from build123d import *

# Parameters (mm, degrees)
BOSS_EXTRUDE1_DEPTH      = 381
BOSS_EXTRUDE1_DEPTH_BACK = 381
SKETCH1_W                = 12.7
SKETCH1_H                = 12.7
SKETCH1_W_2              = 9.525
SKETCH1_H_2              = 9.525


with BuildPart() as part:
    # Sketch1 → Boss-Extrude1 (new, two sides: drawn at the far end of the back side and taken through both)
    with BuildSketch(Plane.XY.offset(-BOSS_EXTRUDE1_DEPTH_BACK)):
        with Locations((323.85, 95.25)):
            Rectangle(SKETCH1_W, SKETCH1_H)
        with Locations((323.85, 95.25)):
            Rectangle(SKETCH1_W_2, SKETCH1_H_2, mode=Mode.SUBTRACT)
    extrude(amount=BOSS_EXTRUDE1_DEPTH + BOSS_EXTRUDE1_DEPTH_BACK)


solid = part.part
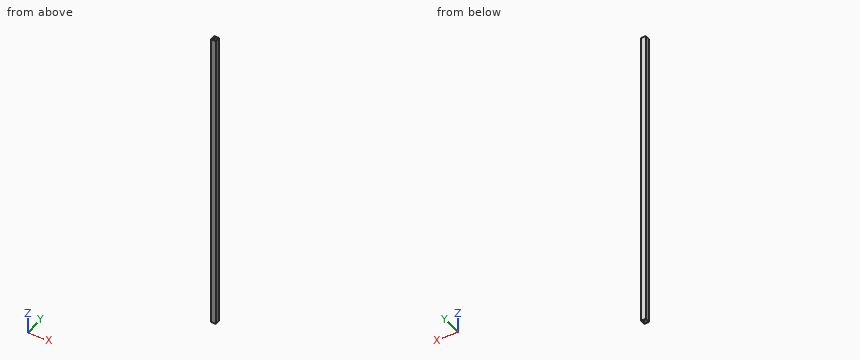
Input: part model. Units: mm. Frame: model coordinates. Give positions to 0.01 mm unless a question says otherwise; leave off trailing zeros. Order: outer loops, then holes, each group sorted by start corner. A loop starts at its lowest first (then second) coordinate and runs counter-clockwise, first axis right, second up. Notation, with made-up numbers: (29.25, 81) - (54.25, 81) arc R11 cw to (54.25, 98) - close; hole circle Ø11 at (4.5, -33). An arc over 180 degrees is marked (long way). Answer as a JSON object with one key per item and string values. Group by question number.
Q1. Cut plane A-A, the plane y = 94. Output: boundary loops of the cut face in (x, z).
Q2. Cut plane C-C, the plane z = 329.5. Output: boundary loops of the cut face in (x, y).
Q3. Line query: probe 1 along Y at (x, z) = (327, 30); probe 2 along X at (y, z) = (98, -84). Output: solid intervals per line, ascending.
Q4. Cut plane B-B, the plane x = 324. Output: boundary loops of the cut face in (y, z).
Results:
{
 "1": {"outline": "(317.5, -381) - (319.09, -381) - (319.09, 381) - (317.5, 381) - close; (328.61, -381) - (330.2, -381) - (330.2, 381) - (328.61, 381) - close"},
 "2": {"outline": "(317.5, 88.9) - (330.2, 88.9) - (330.2, 101.6) - (317.5, 101.6) - close; hole (319.09, 90.49) - (328.61, 90.49) - (328.61, 100.01) - (319.09, 100.01) - close"},
 "3": {"probe 1": "88.9 to 90.49, 100.01 to 101.6", "probe 2": "317.5 to 319.09, 328.61 to 330.2"},
 "4": {"outline": "(88.9, -381) - (90.49, -381) - (90.49, 381) - (88.9, 381) - close; (100.01, -381) - (101.6, -381) - (101.6, 381) - (100.01, 381) - close"}
}
